Read the model definition and answer for the solid it produces. Units are mm, in the model's axes. Face numbers are marked on the shaded views. A direction names the side the tool comes from. Round coordinates to 2 decimals unless told otherwise and drop trailing zeros. Order: outer loops, then holes, each group sorted by start corner. A loop starts at its lowest first (then second) coordinate and runs counter-clockwise, first axis right, second up. Notation, with made-up numbers: M -7.5,52 L 46.5,52 A22 ccw 46.5,74 Z; hole C 40,46 d6. An arc over 180 degrees is marked long. Use one line per item in the form item = value. Start each with the question number.
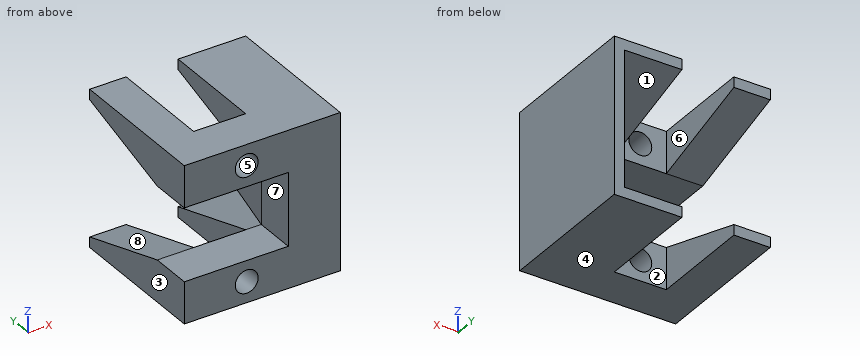
from build123d import *

# Parameters (mm, degrees)
SKETCH_1_W          = 10
SKETCH_1_H          = 4
EXTRUDE_1_DEPTH     = 4
SKETCH_2_W          = 5
SKETCH_2_H          = 11
EXTRUDE_2_DEPTH     = 4
SKETCH_3_W          = 15
SKETCH_3_H          = 4
EXTRUDE_3_DEPTH     = 4
SKETCH_4_R          = 1.1
CUT_EXTRUDE_1_DEPTH = 17.881943016
SKETCH_5_W          = 3.5
SKETCH_5_H          = 4
EXTRUDE_6_DEPTH     = 10
SKETCH_9_W          = 6.5
SKETCH_9_H          = 4
EXTRUDE_7_DEPTH     = 10
SKETCH_11_W         = 5
SKETCH_11_H         = 7
EXTRUDE_8_DEPTH     = 10
CUT_EXTRUDE_3_REACH = 26.29
CHAMFER_2_SIZE      = 10
CHAMFER_2_SIZE2     = 4


with BuildPart() as part:
    # 草图1 → 凸台-拉伸1 (new body)
    with BuildSketch(Plane(origin=(0, 0, 0), x_dir=(1, 0, 0), z_dir=(0, 1, 0))):
        Rectangle(SKETCH_1_W, SKETCH_1_H)
    extrude(amount=EXTRUDE_1_DEPTH)

    # 草图2 → 凸台-拉伸2 (add)
    with BuildSketch(Plane(origin=(0, 4, 0), x_dir=(1, 0, 0), z_dir=(0, 1, 0))):
        with Locations((7.5, -3.5)):
            Rectangle(SKETCH_2_W, SKETCH_2_H)
    extrude(amount=-EXTRUDE_2_DEPTH)

    # 草图3 → 凸台-拉伸3 (add)
    with BuildSketch(Plane(origin=(0, 4, 0), x_dir=(1, 0, 0), z_dir=(0, 1, 0))):
        with Locations((2.5, -11)):
            Rectangle(SKETCH_3_W, SKETCH_3_H)
    extrude(amount=-EXTRUDE_3_DEPTH)

    # 草图4 → 切除-拉伸1 (cut, through all)
    with BuildSketch(Plane(origin=(0, 4, 0), x_dir=(1, 0, 0), z_dir=(0, 1, 0))):
        with Locations(Location((1, -11, 0), (0, 0, 270))):
            Circle(SKETCH_4_R)
        with Locations(Location((1, 0, 0), (0, 0, 270))):
            Circle(SKETCH_4_R)
    extrude(amount=-CUT_EXTRUDE_1_DEPTH, mode=Mode.SUBTRACT)

    # 草图5 → 凸台-拉伸6 (add)
    with BuildSketch(Plane(origin=(0, 4, 0), x_dir=(1, 0, 0), z_dir=(0, 1, 0))):
        with Locations((-3.25, -11)):
            Rectangle(SKETCH_5_W, SKETCH_5_H)
        with Locations((-3.25, 0)):
            Rectangle(SKETCH_5_W, SKETCH_5_H)
    extrude(amount=EXTRUDE_6_DEPTH)

    # 草图9 → 凸台-拉伸7 (add)
    with BuildSketch(Plane(origin=(0, 4, 0), x_dir=(1, 0, 0), z_dir=(0, 1, 0))):
        with Locations((6.75, 0)):
            Rectangle(SKETCH_9_W, SKETCH_9_H)
        with Locations((6.75, -11)):
            Rectangle(SKETCH_9_W, SKETCH_9_H)
    extrude(amount=EXTRUDE_7_DEPTH)

    # 草图11 → 凸台-拉伸8 (add)
    with BuildSketch(Plane(origin=(0, 4, 0), x_dir=(1, 0, 0), z_dir=(0, 1, 0))):
        with Locations((7.5, -5.5)):
            Rectangle(SKETCH_11_W, SKETCH_11_H)
    extrude(amount=EXTRUDE_8_DEPTH)

    # 切除-拉伸3: up to this face of the body (flat: up to its plane)
    cut_extrude_3_end = Plane(part.part.faces().sort_by_distance((5, 7, 5.5))[0])
    # 草图8 → 切除-拉伸3 (cut, up to the picked face)
    with BuildSketch(Plane.ZY.offset(5), mode=Mode.PRIVATE) as cut_extrude_3_sk1:
        Polygon((2, 4), (-1, 14), (2, 14), align=None)
    cut_extrude_3_tool1 = split(extrude(cut_extrude_3_sk1.sketch, amount=-CUT_EXTRUDE_3_REACH, mode=Mode.PRIVATE), bisect_by=cut_extrude_3_end, keep=Keep.BOTH, mode=Mode.PRIVATE)
    # 草图8 → 切除-拉伸3 (cut, up to the picked face)
    with BuildSketch(Plane.ZY.offset(5), mode=Mode.PRIVATE) as cut_extrude_3_sk2:
        Polygon((12, 14), (9, 4), (9, 14), align=None)
    cut_extrude_3_tool2 = split(extrude(cut_extrude_3_sk2.sketch, amount=-CUT_EXTRUDE_3_REACH, mode=Mode.PRIVATE), bisect_by=cut_extrude_3_end, keep=Keep.BOTH, mode=Mode.PRIVATE)
    add(cut_extrude_3_tool1.solids().sort_by(Axis((-5, 10.666667, 1), (1, 0, 0)))[0], mode=Mode.SUBTRACT)
    add(cut_extrude_3_tool2.solids().sort_by(Axis((-5, 10.666667, 10), (1, 0, 0)))[0], mode=Mode.SUBTRACT)

    # 倒角2
    chamfer_2_edges = [part.edges().sort_by_distance(p)[0] for p in [
        (5, 14, 5.5),
    ]]
    chamfer_2_side = [part.faces().sort_by_distance(p)[0] for p in [
        (5, 7.859375, 5.5),
    ]]
    chamfer(chamfer_2_edges, length=CHAMFER_2_SIZE, length2=CHAMFER_2_SIZE2, reference=chamfer_2_side[0])


solid = part.part
Item 1: For a pull along X with two mould halves and no side action, classify the marked faces 1, 2 and 3 as pulls with the +X half, pulls with the -X half, needs draft (parallel to the pull), parting line crosses it, or undercut.
Item 2: Find the intervals of material crossed by L1, parallel to X at y = 2.7, z = 11; L2, parallel to X at y = 11, z = 12; L3, parallel to Y at x = 0.5, z = 12.25, in increasing order. Write a range as [from, to].
Item 3: Section C-C (x = 1) is taken. Write down the section's boundary in (y, z).
Item 4: Section D-D (z = -0.5) is taken. Write down the section's boundary in (x, y).
Item 5: A tool of negligible diameter and unlimited length cuts with its end or side. For the marked faces 4, 5, 6, 7 and 8, from which of +Z, -Z, +X, -X, +Y, -Y can it reach the whole face along a straight path? Write none if from no direction.
Item 6: Section B-B (x = -1.25) is taken. Write down the section's boundary in (y, z), and give its area (3 significant figures).
Item 7: Given P1, Ø4, axis at y = 5.5, z = 6, coming from the -X side; P2, Ø6, axis at x = 8, z = 6.5, coming from the +Y side; P3, Ø3.5, axis at x = 1, z = 11, coming from the +Y side; P4, Ø1.5, axis at y = 6.5, z = 6.5, coming from the -X side, each flat-ended and moving along its own axis, determine where each tip first touches the part or whether it passes through.
Item 8: Section A-A (y = 6.5) is taken. Write down the section's boundary in (x, z).
The answers:
q1.face_1 = needs draft
q1.face_2 = undercut
q1.face_3 = pulls with the -X half
q2.L1 = [-5, -0.1], [2.1, 10]
q2.L2 = [-5, -1.5], [3.5, 10]
q2.L3 = [0, 4]
q3.outline = M 0,-2 L 4,-2 L 4,-1.1 L 0,-1.1 Z; M 0,1.1 L 4,1.1 L 4,2 L 0,2 Z; M 0,9 L 4,9 L 4,9.9 L 0,9.9 Z; M 0,12.1 L 4,12.1 L 4,13 L 0,13 Z
q4.outline = M -5,0 L 0.02,0 L 0.02,4 L -1.5,4 L -1.5,12.33 L -5,12.33 Z; M 1.98,0 L 10,0 L 10,14 L 9,14 L 8.33,12.33 L 3.5,12.33 L 3.5,4 L 1.98,4 Z
q5.face_4 = -Z, +X, -X, +Y, -Y
q5.face_5 = +Y, -Y
q5.face_6 = +Z, -Z, +Y
q5.face_7 = -X, +Y, -Y
q5.face_8 = -X, +Y
q6.outline = M 0,-2 L 4,-2 L 4,2 L 0,2 Z; M 0,9 L 4,9 L 4,13 L 0,13 Z
q6.area = 32.0 mm²
q7.P1 = 5
q7.P2 = 14
q7.P3 = 4
q7.P4 = 5.7
q8.outline = M -5,-2 L -1.5,-2 L -1.5,1.25 L -5,1.25 Z; M -5,9.75 L -1.5,9.75 L -1.5,13 L -5,13 Z; M 3.5,-2 L 10,-2 L 10,13 L 3.5,13 L 3.5,9.75 L 6,9.75 L 6,1.25 L 3.5,1.25 Z
